Design review of the part built by this model. Coordinates are the model's own, in mm. A direction names the side the tool comes from. Round coordinates to 2 decimals unless told otherwise and drop trailing zeros. Write each loop counter-clockwise with the first axis right and the second up, starting at its lowest first coordinate (ties: lowest second). Pieces come first, ordered by that corner, then holes. Notation, with made-up numbers: (21, 7) -> (48, 7) arc R22 ccw to (48, 41) -> close; hole circle Ø3 at (18.25, 20.5). An arc over 180 degrees is marked (long way). One line per question, with ' | ' between items. Start each with the question number.
1) Consider section A-A (z = 7). Give the boundary of the cut face in (x, y).
2) Consider section B-B (y = -18.5). Give the boundary of the cut face in (x, z).
3) For faces 1 (the flat face through (-54.658, -13, 7)), 2 (the flat face through (-13, -13, 11.173)), 3 (the flat face through (-94, -13, 27.083)), 4 (the flat face through (25.4, -13, 37)), 5 (the flat face through (140, -13, 3.295)), list the 3-axis set-ups (+Z, -Z, +X, -X, +Y, -Y) from which the entire face can be reached by the end or side of a thin tool; tool diameter is ignored.
4) For probe 1 along X at (y, z) = (-19.5, 37); probe 2 along X at (y, z) = (-5.25, 4); probe 3 along Z at (x, y) = (-99.5, -13.5), list the stretches that pass through material, from the lowest coordinate up.
5) Insertion check: pin 1 Ø7 at (y, z) = (-9, 5.5) entering from -X; pin 2 Ø1.2 at (y, z) = (-11.5, 13) entering from -X; pin 3 Ø10 at (x, y) = (-44.5, -12) entering from +Z. Each pin has a flat end and moves straight along its axis. Give the tip position at first contact, or say it passes through.
6) Consider section D-D (x = 41). Give the boundary of the cut face in (y, z).
7) Consider section C-C (x = -81.5). Give the boundary of the cut face in (y, z).
```python
from build123d import *

# Parameters (mm, degrees)
F0_W     = 25.4
F0_H     = 6.135838
F0_H_2   = 8.51089
F0_H_3   = 6.558549
F1_DEPTH = 25.4


with BuildPart() as f1:
    # F0 (on Front) → F1 (new body)
    with BuildSketch(Plane.XZ):
        Polygon((0, 34.30898), (-59.153413, 34.30898), (-59.153413, 27.082892), (-59.153413, 15.05862), (-59.153413, 11.173423), (-54.658122, 11.173423), (-29.258122, 11.173423), (4.035674, 11.173423), (29.435674, 11.173423), (84.918008, 11.173423), (84.918008, 34.30898), (25.4, 34.30898), align=None)
        with Locations((12.7, 37.376899)):
            Rectangle(F0_W, F0_H)
        Polygon((-59.153413, 15.05862), (-59.153413, 27.082892), (-129.672574, 27.082892), (-129.672574, 22.232148), (-129.672574, 15.05862), align=None)
        Polygon((127, 34.30898), (84.918008, 34.30898), (84.918008, 11.173423), (127, 11.173423), (127, 3.2947), (152.4, 3.2947), (152.4, 11.173423), (152.4, 34.30898), (152.4, 40.679562), (127, 40.679562), align=None)
        with Locations((-41.958122, 6.917978)):
            Rectangle(F0_W, F0_H_2)
        with Locations((16.735674, 7.894149)):
            Rectangle(F0_W, F0_H_3)
    extrude(amount=F1_DEPTH)


solid = f1.part
```
From the geometry:
1) outline: (-54.66, -25.4) -> (-29.26, -25.4) -> (-29.26, 0) -> (-54.66, 0) -> close; (4.04, -25.4) -> (29.44, -25.4) -> (29.44, 0) -> (4.04, 0) -> close; (127, -25.4) -> (152.4, -25.4) -> (152.4, 0) -> (127, 0) -> close
2) outline: (-129.67, 15.06) -> (-59.15, 15.06) -> (-59.15, 11.17) -> (-54.66, 11.17) -> (-54.66, 2.66) -> (-29.26, 2.66) -> (-29.26, 11.17) -> (4.04, 11.17) -> (4.04, 4.61) -> (29.44, 4.61) -> (29.44, 11.17) -> (127, 11.17) -> (127, 3.29) -> (152.4, 3.29) -> (152.4, 40.68) -> (127, 40.68) -> (127, 34.31) -> (25.4, 34.31) -> (25.4, 40.44) -> (0, 40.44) -> (0, 34.31) -> (-59.15, 34.31) -> (-59.15, 27.08) -> (-129.67, 27.08) -> close
3) face 1: -Z, -X, +Y, -Y | face 2: -Z, +Y, -Y | face 3: +Z, -X, +Y, -Y | face 4: +Z, +Y, -Y | face 5: -Z, +X, +Y, -Y
4) probe 1: x = 0 to 25.4, 127 to 152.4 | probe 2: x = -54.66 to -29.26, 127 to 152.4 | probe 3: z = 15.06 to 27.08
5) pin 1: stops at x = -54.66 | pin 2: stops at x = -59.15 | pin 3: stops at z = 34.31
6) outline: (-25.4, 11.17) -> (0, 11.17) -> (0, 34.31) -> (-25.4, 34.31) -> close
7) outline: (-25.4, 15.06) -> (0, 15.06) -> (0, 27.08) -> (-25.4, 27.08) -> close
